from build123d import *

# Parameters (mm, degrees)
F2_DEPTH = 3
F3_DEPTH = 5


with BuildPart() as f2:
    # F0 (on Top) → F2 (new body)
    with BuildSketch(Plane.XY):
        with BuildLine():
            ThreePointArc((21, 9.96), (20.256051, 11.756051), (18.46, 12.5))
            Line((18.46, 12.5), (-18.46, 12.5))
            ThreePointArc((-18.46, 12.5), (-20.256051, 11.756051), (-21, 9.96))
            Line((-21, 9.96), (-21, -9.96))
            ThreePointArc((-21, -9.96), (-20.256051, -11.756051), (-18.46, -12.5))
            Line((-18.46, -12.5), (18.46, -12.5))
            ThreePointArc((18.46, -12.5), (20.256051, -11.756051), (21, -9.96))
            Line((21, -9.96), (21, 9.96))
        make_face()
    extrude(amount=F2_DEPTH)

    # F1 (on face) → F3 (join)
    with BuildSketch(Plane.XY):
        with BuildLine():
            ThreePointArc((23, 9.96), (21.670265, 13.170265), (18.46, 14.5))
            Line((18.46, 14.5), (-18.46, 14.5))
            ThreePointArc((-18.46, 14.5), (-21.670265, 13.170265), (-23, 9.96))
            Line((-23, 9.96), (-23, -9.96))
            ThreePointArc((-23, -9.96), (-21.670265, -13.170265), (-18.46, -14.5))
            Line((-18.46, -14.5), (18.46, -14.5))
            ThreePointArc((18.46, -14.5), (21.670265, -13.170265), (23, -9.96))
            Line((23, -9.96), (23, 9.96))
        make_face()
        with BuildLine():
            ThreePointArc((18.46, 12.5), (20.256051, 11.756051), (21, 9.96))
            Line((21, 9.96), (21, -9.96))
            ThreePointArc((21, -9.96), (20.256051, -11.756051), (18.46, -12.5))
            Line((18.46, -12.5), (-18.46, -12.5))
            ThreePointArc((-18.46, -12.5), (-20.256051, -11.756051), (-21, -9.96))
            Line((-21, -9.96), (-21, 9.96))
            ThreePointArc((-21, 9.96), (-20.256051, 11.756051), (-18.46, 12.5))
            Line((-18.46, 12.5), (18.46, 12.5))
        make_face(mode=Mode.SUBTRACT)
    extrude(amount=F3_DEPTH)


solid = f2.part
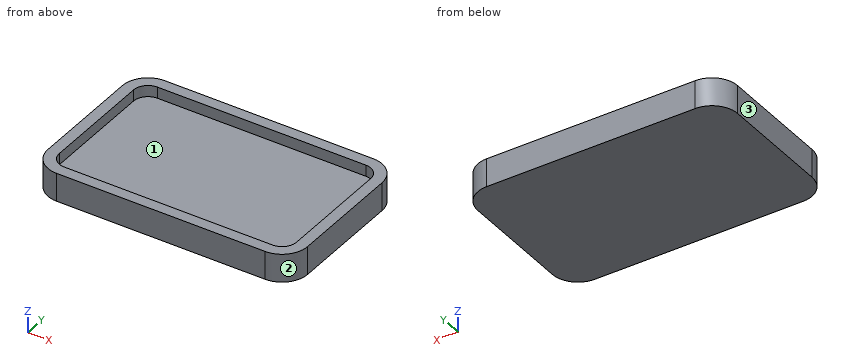
Here's how the part is built. I have some questions about the finished solid (model axes, mm). Face numbers are marked on the shaded views. Coordinates: 2 decimals unless noted, no trailing zeros. Write each loop counter-clockwise with the first axis right and the second up, starting at its lowest first coordinate (ties: lowest second). Pieces come first, ordered by that corner, then holes.
1) If we section it at C-C (y = 6): List the corners of the cut face in (x, z) for me, plus the area to 3 significant figures.
Filled in:
outline: (-23, 0) - (23, 0) - (23, 5) - (21, 5) - (21, 3) - (-21, 3) - (-21, 5) - (-23, 5) - close
area: 146 mm2
2) I'm going to push a flat-ended pin straight in: pin 1 (12.5 mm diameter, centred on x = 0.5, y = 2, fed in from +Z). Where does the tip first touch, or does it pass through?
Filled in:
pin 1: stops at z = 3
3) Thinking about a two-plate mould opening in Y: for the marked faces 1, 2 and 3, which applies, +Y half, -Y half, draft (parallel to the pull), parting line (faces both ways), or undercut?
Filled in:
face 1: undercut
face 2: -Y half
face 3: draft
4) If I drill on line 1 (X direction, y = -0.25, z = 4.5); line 2 (Y direction, x = 0, z = 3.95); line 3 (Z direction, x = 9, y = -11), over which ranges is the centre line in solid material (lowest first)?
Filled in:
line 1: x = -23 to -21, 21 to 23
line 2: y = -14.5 to -12.5, 12.5 to 14.5
line 3: z = 0 to 3
5) If we section it at A-A (z = 4.1): List the corners of the cut face in (x, y) for me.
Filled in:
outline: (-23, -9.96) arc R4.54 ccw to (-18.46, -14.5) - (18.46, -14.5) arc R4.54 ccw to (23, -9.96) - (23, 9.96) arc R4.54 ccw to (18.46, 14.5) - (-18.46, 14.5) arc R4.54 ccw to (-23, 9.96) - close; hole (-21, -9.96) arc R2.54 ccw to (-18.46, -12.5) - (18.46, -12.5) arc R2.54 ccw to (21, -9.96) - (21, 9.96) arc R2.54 ccw to (18.46, 12.5) - (-18.46, 12.5) arc R2.54 ccw to (-21, 9.96) - close
6) If we section it at B-B (x = -2): List the corners of the cut face in (y, z) for me, plus the area to 3 significant figures.
Filled in:
outline: (-14.5, 0) - (14.5, 0) - (14.5, 5) - (12.5, 5) - (12.5, 3) - (-12.5, 3) - (-12.5, 5) - (-14.5, 5) - close
area: 95.0 mm2
